Autodesk Inventor part; units mm, degrees
ref_plane "YZ Plane" through (0, 0, 0) normal (1, 0, 0) x (0, 1, 0)
ref_plane "XZ Plane" through (0, 0, 0) normal (0, 1, 0) x (-1, 0, 0)
ref_plane "XY Plane" through (0, 0, 0) normal (0, 0, 1) x (1, 0, 0)
sketch "Sketch1" plane through (0, 0, 0) normal (1, 0, 0) x (0, 1, 0)
  line L0 (0, -15) -> (0, 62)
  line L1 (0, -4) -> (15, -4)
  line L2 (15, -4) -> (15, 0)
  line L3 (15, 0) -> (12.5, 0)
  line L4 (12.5, 0) -> (12.5, 146)
  line L5 (12.5, 146) -> (0, 146)
  line L6 (0, 146) -> (0, -4)
  point P0 (0, 0)
  dimension "d28" = 4
  dimension "d29" = 30
  dimension "d31" = 25
  dimension "d33" = 150
revolve "Revolution1" add sketch "Sketch1" angle 360 about axis through (0, 0, -10) along (0, 0, 1)
sketch "Sketch2" plane through (0, 0, 0) normal (1, 0, 0) x (0, 1, 0)
  line L0 (12.5, 146) -> (12.5, 0) construction
  line L1 (-12.5, 0) -> (12.5, 0) construction
  line L2 (12.5, 0) -> (12.3, 0)
  line L3 (12, 0.3) -> (12, 0.9)
  line L4 (12.3, 1.2) -> (12.5, 1.2)
  line L5 (12.5, 1.2) -> (12.5, 0)
  arc A0 (12.3, 1.2) -> (12, 0.9) centre (12.3, 0.9) ccw
  arc A1 (12, 0.3) -> (12.3, 0) centre (12.3, 0.3) ccw
  line L6 (0, -10.2746) -> (0, 61.2124)
  point P0 (0, 0)
  dimension "d45" = 0.3
  dimension "d46" = 1.2
  dimension "d47" = 0.5
revolve "Revolution2" cut sketch "Sketch2" angle 360 about axis through (0, 0, -10) along (0, 0, 1)
chamfer "Chamfer1" distance 0.5 angle 45 3 edges at (0, -12.5, 146) (0, -15, 0) (0, -15, -4)
equation "\"d28\" = H_"
equation "\"d29\" = D"
equation "\"d31\" = d_"
equation "\"d33\" = L"
equation "\"d_\" = 25"
equation "\"L\" = 150"
equation "\"D\" = 30"
equation "\"H_\" = 4"
properties part number "M-RPN25x150" material "SUJ 2"
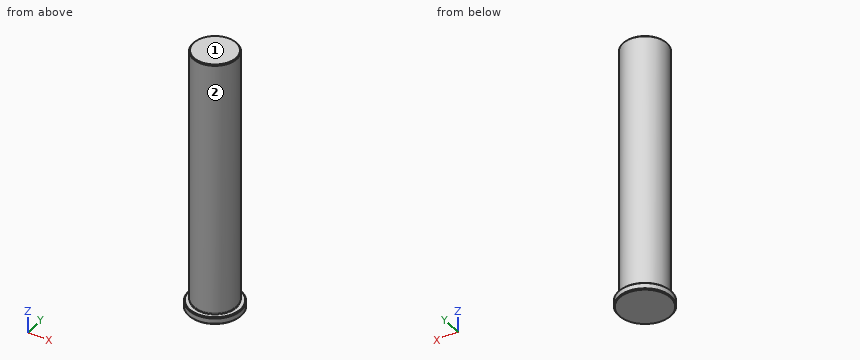
Can you work these out from the model? Positions are in its coordinate system, mm. Face numbers are marked on the shaded views. A direction names the side the tool comes from. Give positions to 0.01 mm unless a question says otherwise; leave off trailing zeros. Loops run counter-clockwise (first coordinate to the right, second up) from the corner with the lowest first, then second, coordinate; pieces in that order, holes last. Notation, with made-up numbers: (55, 12) - (78, 12) arc R23 ccw to (78, 31) - close; hole circle Ø10 at (23, -27). An arc over 180 degrees is marked (long way). Return JSON: item names as keys, results as strings.
1. If I drill on line 1 (Z direction, x = -12.75, y = 6); line 2 (Z direction, x = -7.25, y = 9.75); line 3 (X direction, y = 10, z = 85.5), over which ranges is the centre line in solid material (lowest first)?
Output values:
{"line 1": "z = -4 to 0", "line 2": "z = -4 to 0.04, 1.16 to 145.85", "line 3": "x = -7.5 to 7.5"}
2. I'm going to push flat-ended pins straight in: pin 1 Ø2 at (y, z) = (8.5, 77) entering from +X; pin 2 Ø8 at (x, z) = (-8.5, 30) entering from +Y; pin 3 Ø5 at (x, z) = (-1, 25) entering from -Y. Where does each tip first touch, or does it pass through?
Output values:
{"pin 1": "stops at x = 10", "pin 2": "stops at y = 11.66", "pin 3": "stops at y = -12.5"}
3. For the marked faces 1 and 2, which set-ups out of +Z, -Z, +X, -X, +Y, -Y let a thin tool reach every point of the face, with its end or its side?
Output values:
{"face 1": "+Z, +X, -X, +Y, -Y", "face 2": "+Z"}
4. I want a section at A-A on y = 0. Please give me the cut outline in (x, z), and give its area (3 significant figures).
Output values:
{"outline": "(-15, -3.5) - (-14.5, -4) - (14.5, -4) - (15, -3.5) - (15, -0.5) - (14.5, 0) - (12.3, 0) arc R0.3 cw to (12, 0.3) - (12, 0.9) arc R0.3 cw to (12.3, 1.2) - (12.5, 1.2) - (12.5, 145.5) - (12, 146) - (-12, 146) - (-12.5, 145.5) - (-12.5, 1.2) - (-12.3, 1.2) arc R0.3 cw to (-12, 0.9) - (-12, 0.3) arc R0.3 cw to (-12.3, 0) - (-14.5, 0) - (-15, -0.5) - close", "area": "3,770 mm²"}
5. I want a section at C-C on z = 65.5. Please give me the cut outline in (x, y), and give its area (3 significant figures).
Output values:
{"outline": "circle Ø25 at (0, 0)", "area": "491 mm²"}
